from build123d import *

# Parameters (mm, degrees)
F2_SIZE  = 2
F4_DEPTH = 25
F5_R     = 1


# Not quite as in the source:
# - a fillet or chamfer that OpenCascade refuses, or shapes differently, is made with other operations: its cross-section is extruded or revolved along the edge and cut away or added


with BuildPart() as f1:
    # F0 (on Front) → F1 (revolve)
    with BuildSketch(Plane.XZ):
        with BuildLine():
            Line((4.2, 22.5), (4.2, 0))
            Line((4.2, 0), (19.2955706467, 0))
            Line((19.2955706467, 0), (21.5, 2.499420478))
            Line((21.5, 2.499420478), (20.5, 2.499420478))
            Line((20.5, 2.499420478), (10.1050306112, 2.499420478))
            ThreePointArc((10.1050306112, 2.499420478), (5.8563757844, 11.7216769606), (6.0455347411, 21.8737851828))
            Line((6.0455347411, 21.8737851828), (5.5262264796, 22.5))
            Line((5.5262264796, 22.5), (4.2, 22.5))
        make_face()
    revolve(axis=Axis((0, 0, 11.7304213345), (0, 0, 1)))

    # F2
    f2_edges = [f1.edges().sort_by_distance(p)[0] for p in [
        (-4.2, 0, 0),
    ]]
    chamfer(f2_edges, length=F2_SIZE)

    # F3 (on face) → F4 (cut)
    with BuildSketch(Plane(origin=(0, 0, 0), x_dir=(1, 0, 0), z_dir=(0, 0, -1))):
        with BuildLine():
            ThreePointArc((14.132025682, -3.23120262), (14.6068235272, -3.3834984393), (15.104538526, -3.4136113971))
            ThreePointArc((15.104538526, -3.4136113971), (18.3046103696, 0), (15.104538526, 3.4136113971))
            ThreePointArc((15.104538526, 3.4136113971), (14.6068235272, 3.3834984393), (14.132025682, 3.23120262))
            Line((14.132025682, 3.23120262), (7.1852975525, 0))
            Line((7.1852975525, 0), (14.132025682, -3.23120262))
        make_face()
        with BuildLine():
            ThreePointArc((12.2776564756, 7.7080459076), (12.7210786582, 7.9360892771), (13.0943093857, 8.2667338512))
            ThreePointArc((13.0943093857, 8.2667338512), (12.9433141193, 12.9433141193), (8.2667338512, 13.0943093857))
            ThreePointArc((8.2667338512, 13.0943093857), (7.9360892771, 12.7210786582), (7.7080459076, 12.2776564756))
            Line((7.7080459076, 12.2776564756), (5.0807726242, 5.0807726242))
            Line((5.0807726242, 5.0807726242), (12.2776564756, 7.7080459076))
        make_face()
        with BuildLine():
            ThreePointArc((3.23120262, 14.132025682), (3.3834984393, 14.6068235272), (3.4136113971, 15.104538526))
            ThreePointArc((3.4136113971, 15.104538526), (0, 18.3046103696), (-3.4136113971, 15.104538526))
            ThreePointArc((-3.4136113971, 15.104538526), (-3.3834984393, 14.6068235272), (-3.23120262, 14.132025682))
            Line((-3.23120262, 14.132025682), (0, 7.1852975525))
            Line((0, 7.1852975525), (3.23120262, 14.132025682))
        make_face()
        with BuildLine():
            ThreePointArc((-7.7080459076, 12.2776564756), (-7.9360892771, 12.7210786582), (-8.2667338512, 13.0943093857))
            ThreePointArc((-8.2667338512, 13.0943093857), (-12.9433141193, 12.9433141193), (-13.0943093857, 8.2667338512))
            ThreePointArc((-13.0943093857, 8.2667338512), (-12.7210786582, 7.9360892771), (-12.2776564756, 7.7080459076))
            Line((-12.2776564756, 7.7080459076), (-5.0807726242, 5.0807726242))
            Line((-5.0807726242, 5.0807726242), (-7.7080459076, 12.2776564756))
        make_face()
        with BuildLine():
            ThreePointArc((-14.132025682, 3.23120262), (-14.6068235272, 3.3834984393), (-15.104538526, 3.4136113971))
            ThreePointArc((-15.104538526, 3.4136113971), (-18.3046103696, 0), (-15.104538526, -3.4136113971))
            ThreePointArc((-15.104538526, -3.4136113971), (-14.6068235272, -3.3834984393), (-14.132025682, -3.23120262))
            Line((-14.132025682, -3.23120262), (-7.1852975525, 0))
            Line((-7.1852975525, 0), (-14.132025682, 3.23120262))
        make_face()
        with BuildLine():
            ThreePointArc((-12.2776564756, -7.7080459076), (-12.7210786582, -7.9360892771), (-13.0943093857, -8.2667338512))
            ThreePointArc((-13.0943093857, -8.2667338512), (-12.9433141193, -12.9433141193), (-8.2667338512, -13.0943093857))
            ThreePointArc((-8.2667338512, -13.0943093857), (-7.9360892771, -12.7210786582), (-7.7080459076, -12.2776564756))
            Line((-7.7080459076, -12.2776564756), (-5.0807726242, -5.0807726242))
            Line((-5.0807726242, -5.0807726242), (-12.2776564756, -7.7080459076))
        make_face()
        with BuildLine():
            ThreePointArc((-3.23120262, -14.132025682), (-3.3834984393, -14.6068235272), (-3.4136113971, -15.104538526))
            ThreePointArc((-3.4136113971, -15.104538526), (0, -18.3046103696), (3.4136113971, -15.104538526))
            ThreePointArc((3.4136113971, -15.104538526), (3.3834984393, -14.6068235272), (3.23120262, -14.132025682))
            Line((3.23120262, -14.132025682), (0, -7.1852975525))
            Line((0, -7.1852975525), (-3.23120262, -14.132025682))
        make_face()
        with BuildLine():
            ThreePointArc((7.7080459076, -12.2776564756), (7.9360892771, -12.7210786582), (8.2667338512, -13.0943093857))
            ThreePointArc((8.2667338512, -13.0943093857), (12.9433141193, -12.9433141193), (13.0943093857, -8.2667338512))
            ThreePointArc((13.0943093857, -8.2667338512), (12.7210786582, -7.9360892771), (12.2776564756, -7.7080459076))
            Line((12.2776564756, -7.7080459076), (5.0807726242, -5.0807726242))
            Line((5.0807726242, -5.0807726242), (7.7080459076, -12.2776564756))
        make_face()
    extrude(amount=-F4_DEPTH, mode=Mode.SUBTRACT)

    # F5
    f5_edges = [f1.edges().sort_by_distance(p)[0] for p in [
        (-6.045535, 0, 21.873785),
    ]]
    fillet(f5_edges, radius=F5_R)

    # F6: fillet of radius 1 on 1 edges, made by hand

    # F6_s1 → F6_t2 (revolve, cut)
    with BuildSketch(Plane.XZ):
        with BuildLine():
            ThreePointArc((5.7271677505, 22.2576998048), (5.4226307234, 22.4374699475), (5.0745644975, 22.5))
            Line((5.0745644975, 22.5), (5.5262264796, 22.5))
            ThreePointArc((5.5262264796, 22.5), (5.6266952661, 22.3788483691), (5.7271677505, 22.2576998048))
        make_face()
    revolve(axis=Axis((0, 0, 22.5), (0, 0, 1)), mode=Mode.SUBTRACT)

    # F7: chamfer of 1 on 1 edges, made by hand

    # F7_s1 → F7_t2 (revolve, cut)
    with BuildSketch(Plane.XZ):
        Polygon((5.2, 22.5), (4.2, 21.5), (4.2, 22.5), align=None)
    revolve(axis=Axis((0, 0, 22.5), (0, 0, 1)), mode=Mode.SUBTRACT)


solid = f1.part
Read the model definition and answer for the solid it produces. Units are mm, in the model's axes. A direction names the side the tool comes from. Round coordinates to 2 decimals unless told otherwise and drop trailing zeros. Loops run counter-clockwise (first coordinate to the right, second up) from the corner with the lowest first, then second, coordinate; pieces in that order, holes last.
Q1. Section A-A on z = 16.5 is taken. Write down the section's boundary in (x, y), and give its area (3 significant figures).
Q2. Determine the mould class of faces 4 (the face through (4.6, 4.6, 0)), 5 (the face through (-4.213, -18.971, 0.156)), 6 (the face through (7.829, -6.084, 2.028)) for opening direction X: released by +X, released by -X, zero draft, split by the parting line, or undercut.
Q3. Consider probe 1 along Z at (x, y) = (17.5, 7.5); probe 2 along X at (y, z) = (0.5, 8); probe 3 along X at (y, z) = (1, 8). Determine where each line is inside the solid, lowest interval first.
Q4. Each of these flat-tipped pins is pushed along its axis until it touches: pin 1 (8 mm diameter, centred on x = 4, z = 17, fed in from -Y); pin 2 (1.5 mm diameter, centred on y = 0.5, z = 11, fed in from +X); pin 3 (10 mm diameter, centred on y = 4.5, z = 11, fed in from +X); pin 4 (7.5 mm diameter, centred on x = 0, y = 0, fed in from -Z). Where does it stop, or does it pass through?
Q5. Which of the six approach directions +Z, -Z, +X, -X, +Y, -Y give full straight-line access (tool end or side, diameter ignored) to faces 1 (the face through (4.13, 1.3, 1.87)), 2 (the face through (-18.304, -0.072, 1.232)), 3 (the face through (4.5, -9.3, 2.499))?
Q6. Section B-B on y = -11 is taken. Give the number of separate pieces and of enclosed holes in the cut face, and give its area (3 significant figures).
Output:
1. outline: circle Ø10.75 at (0, 0); hole circle Ø8.4 at (0, 0)
1. area: 35.3 mm2
2. face 4: zero draft
2. face 5: split by the parting line
2. face 6: undercut
3. probe 1: z = 0 to 2.5
3. probe 2: x = -6.96 to -4.17, 4.17 to 6.96
3. probe 3: x = -6.9 to -4.08, 4.08 to 6.9
4. pin 1: stops at y = -5.52
4. pin 2: stops at x = 6.2
4. pin 3: stops at x = 7.28
4. pin 4: passes through
5. face 1: -Z
5. face 2: +Z, -Z
5. face 3: +Z
6. separate pieces: 4
6. enclosed holes: 0
6. area: 43.6 mm2
